from build123d import *

# Parameters (mm, degrees)
SKETCH003_W  = 1.2
SKETCH003_H  = 5.5
SKETCH_R     = 3.5
PAD_DEPTH    = 0.44
SKETCH001_R  = 2.2
PAD001_DEPTH = 1.2
FILLET_R     = 1
POCKET_DEPTH = 1
CHAMFER_SIZE = 0.3


with BuildPart() as screw_body:
    # Sketch003 → Revolution (revolve)
    with BuildSketch(Plane.XZ):
        with Locations((0.6, -2.75)):
            Rectangle(SKETCH003_W, SKETCH003_H)
    revolve(axis=Axis((0, 0, 0), (0, 0, 1)))


with BuildPart() as chamfer_body:
    # Sketch → Pad (new body)
    with BuildSketch(Plane.XY):
        Circle(SKETCH_R)
    extrude(amount=PAD_DEPTH)

    # Sketch001 → Pad001 (new body)
    with BuildSketch(Plane.XY.offset(0.44)):
        Circle(SKETCH001_R)
    extrude(amount=PAD001_DEPTH)

    # Fillet
    fillet_edges = [chamfer_body.edges().sort_by_distance(p)[0] for p in [
        (-2.2, 0, 1.64),
    ]]
    fillet(fillet_edges, radius=FILLET_R)

    # Sketch002 → Pocket (cut)
    with BuildSketch(Plane.XY.offset(1.64)):
        with BuildLine():
            Line((-0.3, 1.175), (0.3, 1.175))
            Line((0.3, 1.175), (0.3, 0.8))
            ThreePointArc((0.3, 0.8), (0.446447, 0.446447), (0.8, 0.3))
            Line((0.8, 0.3), (1.175, 0.3))
            Line((1.175, 0.3), (1.175, -0.3))
            Line((1.175, -0.3), (0.8, -0.3))
            ThreePointArc((0.8, -0.3), (0.446447, -0.446447), (0.3, -0.8))
            Line((0.3, -0.8), (0.3, -1.175))
            Line((0.3, -1.175), (-0.3, -1.175))
            Line((-0.3, -1.175), (-0.3, -0.8))
            ThreePointArc((-0.3, -0.8), (-0.446447, -0.446447), (-0.8, -0.3))
            Line((-0.8, -0.3), (-1.175, -0.3))
            Line((-1.175, -0.3), (-1.175, 0.3))
            Line((-1.175, 0.3), (-0.8, 0.3))
            ThreePointArc((-0.8, 0.3), (-0.446447, 0.446447), (-0.3, 0.8))
            Line((-0.3, 0.8), (-0.3, 1.175))
        make_face()
    extrude(amount=-POCKET_DEPTH, mode=Mode.SUBTRACT)

    # Fusion: union screw-body
    add(screw_body.part)

    # Chamfer
    chamfer_edges = [chamfer_body.edges().sort_by_distance(p)[0] for p in [
        (-1.2, 0, 0),
    ]]
    chamfer(chamfer_edges, length=CHAMFER_SIZE)


solid = chamfer_body.part
The listing builds one solid part. Answer for the finished solid, in the listing's coordinates (mm). A direction names the side the tool comes from. Give positions to 0.01 mm unless a question says otherwise; leave off trailing zeros. Order: outer loops, then holes, each group sorted by start corner. A loop starts at its lowest first (then second) coordinate and runs counter-clockwise, first axis right, second up. Notation, with made-up numbers: (22.5, -39.5) - (74.5, -39.5) arc R16 cw to (74.5, -9.5) - close; hole circle Ø2 at (7, 46). An arc over 180 degrees is marked (long way). Use one line per item in the form item = value.
1) Find section A-A on y = 0. Determine the outline of the cut face in (x, z) (3 decimals).
Verdict:
outline = (-3.5, 0) - (-1.5, 0) - (-1.2, -0.3) - (-1.2, -5.5) - (1.2, -5.5) - (1.2, -0.3) - (1.5, 0) - (3.5, 0) - (3.5, 0.44) - (2.2, 0.44) - (2.2, 0.64) arc R1 ccw to (1.2, 1.64) - (1.175, 1.64) - (1.175, 0.64) - (-1.175, 0.64) - (-1.175, 1.64) - (-1.2, 1.64) arc R1 ccw to (-2.2, 0.64) - (-2.2, 0.44) - (-3.5, 0.44) - close
2) The mould has two halves that part along X. Classify faces 1 (the cylindrical face through (0.65, 1.01, -2.86)), 2 (the flat face through (0, 0, 0.64)), 3 (the flat face through (-2, -2, 0.44)): released by +X, released by -X, zero draft, split by the parting line, or undercut.
Verdict:
face_1 = split by the parting line
face_2 = undercut
face_3 = zero draft
3) For faces 4 (the flat face through (0.6, -0.6, 1.64)), 5 (the flat face through (0, -2, 0)), determine the directions among +Z, -Z, +X, -X, +Y, -Y from which every point of the face is accessible in a straight line to the end or side of a thin tool.
Verdict:
face_4 = +Z, +X, -X, +Y, -Y
face_5 = -Z
4) Consider probe 1 along Z at (x, y) = (1, -2.75); probe 2 along Y at (x, z) = (0, -2.5); probe 3 along Z at (x, y) = (-0.75, 0). Determine where each line is inside the solid, lowest interval first. Write a range as [from, to].
Verdict:
probe_1 = [0, 0.44]
probe_2 = [-1.2, 1.2]
probe_3 = [-5.5, 0.64]
5) Find section D-D on x = 2.5. Determine the outline of the cut face in (y, z).
Verdict:
outline = (-2.45, 0) - (2.45, 0) - (2.45, 0.44) - (-2.45, 0.44) - close
6) Each of these flat-tipped pins is pushed along its axis until it touches: pin 1 (0.5 mm diameter, centred on y = 0, z = 1.5, fed in from -X); pin 2 (0.5 mm diameter, centred on x = 0, z = 1.5, fed in from -Y); pin 3 (1 mm diameter, centred on x = 0.5, z = -1.5, fed in from +Y). Where does it stop, or does it pass through?
Verdict:
pin_1 = -1.99
pin_2 = -1.99
pin_3 = 1.2
7) Find section C-C on z = -4.25. Determine the outline of the cut face in (x, y), and give its area (3 significant figures).
Verdict:
outline = circle Ø2.4 at (0, 0)
area = 4.52 mm^2
